```python
from build123d import *

# Parameters (mm, degrees)
F0_W     = 70
F0_H     = 300
F1_DEPTH = 35
F3_DEPTH = 35.001
F6_DEPTH = 17.5
F8_DEPTH = 35.001
F9_DEPTH = 17.5


with BuildPart() as f1:
    # F0 (on Front) → F1 (new body)
    with BuildSketch(Plane.XZ):
        with Locations((35, 150)):
            Rectangle(F0_W, F0_H)
    extrude(amount=F1_DEPTH)

    # F2 (on face) → F3 (cut, through all)
    with BuildSketch(Plane(origin=(0, 0, 0), x_dir=(-1, 0, 0), z_dir=(0, 1, 0))):
        Polygon((-26, 300), (-70, 300), (-70, 256), align=None)
        Polygon((0, 300), (-26, 300), (0, 272), align=None)
    extrude(amount=-F3_DEPTH, mode=Mode.SUBTRACT)

    # F5 (on face) → F6 (cut)
    with BuildSketch(Plane(origin=(0, 0, 0), x_dir=(-1, 0, 0), z_dir=(0, 1, 0))):
        Polygon((-70, 256), (-70, 186), (0, 256), (0, 272), (-26, 300), align=None)
    extrude(amount=-F6_DEPTH, mode=Mode.SUBTRACT)

    # F7 (on face) → F8 (cut, through all)
    with BuildSketch(Plane(origin=(0, 0, 0), x_dir=(-1, 0, 0), z_dir=(0, 1, 0))):
        Polygon((0, 0), (0, 28), (-26, 0), align=None)
    extrude(amount=-F8_DEPTH, mode=Mode.SUBTRACT)

    # F7 (on face) → F9 (cut)
    with BuildSketch(Plane(origin=(0, 0, 0), x_dir=(-1, 0, 0), z_dir=(0, 1, 0))):
        Polygon((0, 98), (-70, 48.732314), (-70, 0), (-26, 0), (0, 28), align=None)
    extrude(amount=-F9_DEPTH, mode=Mode.SUBTRACT)


solid = f1.part
```
Read the model definition and answer for the solid it produces. Units are mm, in the model's axes. A direction names the side the tool comes from. Coordinates: 2 decimals unless noted, no trailing zeros. Loops run counter-clockwise (first coordinate to the right, second up) from the corner with the lowest first, then second, coordinate; pieces in that order, holes last. Notation, with made-up numbers: (30.25, 7.5) - (59.25, 7.5) arc R22 ccw to (59.25, 45.5) - close; hole circle Ø6 at (68, -22.5). An arc over 180 degrees is marked (long way). Answer in a Markdown table with one row per item.
1. Straight lines are drawn through the part: line 1 (Y direction, x = 5, z = 275.5); line 2 (X direction, y = -4.5, z = 218); line 3 (Z direction, x = 51.5, y = -30). For each, find the intervals that lie inside material, in ascending order.
Conclusion:
| item | result |
|---|---|
| line 1 | y = -35 to -17.5 |
| line 2 | x = 0 to 38 |
| line 3 | z = 0 to 274.5 |
2. Find section C-C, the plane y = -28. Write down the section's boundary in (x, z).
Conclusion:
| item | result |
|---|---|
| outline | (0, 28) - (26, 0) - (70, 0) - (70, 256) - (26, 300) - (0, 272) - close |
3. Given pin 1 (8 mm diameter, centred on x = 13.5, y = -19, fed in from +Z); pin 2 (6 mm diameter, centred on x = 45.5, y = -11.5, fed in from -Z); pin 3 (21 mm diameter, centred on x = 46, z = 256.5, fed in from +Y), each flat-ended and moving along its own axis, determine where each tip first touches the part or whether it passes through.
Conclusion:
| item | result |
|---|---|
| pin 1 | stops at z = 290.85 |
| pin 2 | stops at z = 63.86 |
| pin 3 | stops at y = -17.5 |
4. Which of the six approach directions +Z, -Z, +X, -X, +Y, -Y give full straight-line access (tool end or side, diameter ignored) to faces 1 (the face through (70, -21, 126)), 2 (the face through (35, -9, 221)), 3 (the face through (35, -17.5, 39))?
Conclusion:
| item | result |
|---|---|
| face 1 | +Z, -Z, +X, +Y, -Y |
| face 2 | +Z, +X, +Y |
| face 3 | -Z, -X, +Y |
5. Find section A-A, the plane z = 249. Write down the section's boundary in (x, y), then the cut area to 3 significant figures.
Conclusion:
| item | result |
|---|---|
| outline | (0, -35) - (70, -35) - (70, -17.5) - (7, -17.5) - (7, 0) - (0, 0) - close |
| area | 1,350 mm² |
6. Find section D-D, the plane x = 65.5. Write down the section's boundary in (y, z).
Conclusion:
| item | result |
|---|---|
| outline | (-35, 0) - (-17.5, 0) - (-17.5, 51.9) - (0, 51.9) - (0, 190.5) - (-17.5, 190.5) - (-17.5, 260.5) - (-35, 260.5) - close |
7. Find section B-B, the plane x = 40. Write down the section's boundary in (y, z), then the cut area to 3 significant figures.
Conclusion:
| item | result |
|---|---|
| outline | (-35, 0) - (-17.5, 0) - (-17.5, 69.85) - (0, 69.85) - (0, 216) - (-17.5, 216) - (-17.5, 286) - (-35, 286) - close |
| area | 7,560 mm² |
